```python
from build123d import *

# Parameters (mm, degrees)
F0_W     = 279.4
F0_H     = 25.4
F1_DEPTH = 25.4
F2_R     = 6.35
F3_DEPTH = 25.4
F4_W     = 152.4
F4_H     = 6.35
F5_DEPTH = 25.401


with BuildPart() as f1:
    # F0 (on Top) → F1 (new body)
    with BuildSketch(Plane.XY):
        Rectangle(F0_W, F0_H)
        with BuildLine():
            Line((139.7, 12.7), (139.7, -12.7))
            ThreePointArc((139.7, -12.7), (152.4, 0), (139.7, 12.7))
        make_face()
        with BuildLine():
            ThreePointArc((-139.7, 12.7), (-152.4, 0), (-139.7, -12.7))
            Line((-139.7, -12.7), (-139.7, 12.7))
        make_face()
    extrude(amount=F1_DEPTH)

    # F2 (on face) → F3 (cut, through all)
    with BuildSketch(Plane.XY.offset(25.4)):
        with Locations((-139.7, 0)):
            Circle(F2_R)
        with Locations((139.7, 0)):
            Circle(F2_R)
    extrude(amount=-F3_DEPTH, mode=Mode.SUBTRACT)

    # F4 (on face) → F5 (cut, through all)
    with BuildSketch(Plane.XZ.offset(12.7)):
        with Locations((-203.2, 22.225)):
            Rectangle(F4_W, F4_H)
        with Locations((-203.2, 3.175)):
            Rectangle(F4_W, F4_H)
        with Locations((203.2, 22.225)):
            Rectangle(F4_W, F4_H)
        with Locations((203.2, 3.175)):
            Rectangle(F4_W, F4_H)
    extrude(amount=-F5_DEPTH, mode=Mode.SUBTRACT)


solid = f1.part
```
Could you check a few things on this model? Use its own coordinates, in mm. A direction names the side the tool comes from. Round coordinates to 2 decimals unless told otherwise and drop trailing zeros. Loops run counter-clockwise (first coordinate to the right, second up) from the corner with the lowest first, then second, coordinate; pieces in that order, holes last.
Q1. Thinking about a two-plate mould opening in Y: for faces 1 (the flat face through (-2, 12.7, 13)), 2 (the cylindrical face through (-146.044, 0.279, 12.789)), 3 (the cylindrical face through (133.356, 0.279, 12.789)), 4 (the flat face through (-127, 0, 22)), which applies, pulls with the +Y half, pulls with the -Y half, needs draft (parallel to the pull), parting line crosses it, or undercut?
Q2. I want a section at A-A (y = 0). Write out the boundary of the cut face in (x, z).
Q3. On a 3-axis mill with a long thin cutter (end or side, diameter ignored), from which of +Z, -Z, +X, -X, +Y, -Y can I reach the whole of each face in a straight line? I mean faces 5 (the flat face through (-137, -6, 6.35)), 6 (the flat face through (-137, -6, 19.05)), 7 (the flat face through (133.9, -3, 6.35)), 8 (the flat face through (133.9, -3, 19.05)), 9 (the flat face through (-2, 0, 25.4)). Say none if no direction works.
Q4. For P1, Ø12.5, axis at x = -146, y = 1.5, coming from the -Z side; P2, Ø1.9, axis at y = 5.5, z = 23, coming from the +X side; P3, Ø7, axis at y = -4.5, z = 2, coming from the -X side; P4, Ø11.5, axis at x = -139.7, y = 0, coming from the +Z side, each with a flat end and sliding along its axis, tell me the tip position at first contact or that it passes through.
Q5. Please list where these lines run through material, in increasing order: L1, parallel to X at y = -0.5, z = 9.5; L2, parallel to Y at x = 139.7, z = 9.5; L3, parallel to X at y = -1.25, z = 12.5.
Answer below:
1. face 1: pulls with the +Y half
1. face 2: undercut
1. face 3: undercut
1. face 4: needs draft
2. outline: (-152.4, 6.35) - (-146.05, 6.35) - (-146.05, 19.05) - (-152.4, 19.05) - close; (-133.35, 6.35) - (-127, 6.35) - (-127, 0) - (127, 0) - (127, 6.35) - (133.35, 6.35) - (133.35, 19.05) - (127, 19.05) - (127, 25.4) - (-127, 25.4) - (-127, 19.05) - (-133.35, 19.05) - close; (146.05, 6.35) - (152.4, 6.35) - (152.4, 19.05) - (146.05, 19.05) - close
3. face 5: -Z, -X, +Y, -Y
3. face 6: +Z, -X, +Y, -Y
3. face 7: -Z, +X, +Y, -Y
3. face 8: +Z, +X, +Y, -Y
3. face 9: +Z, +X, -X, +Y, -Y
4. P1: stops at z = 6.35
4. P2: stops at x = 127
4. P3: stops at x = -127
4. P4: passes through
5. L1: x = -152.39 to -146.03, -133.37 to 133.37, 146.03 to 152.39
5. L2: y = -12.7 to -6.35, 6.35 to 12.7
5. L3: x = -152.34 to -145.93, -133.47 to 133.47, 145.93 to 152.34
